Input: part model. Units: mm. Frame: model coordinates. Round coordinates to 2 decimals unless told otherwise and drop trailing zeros. Write each loop counter-clockwise with the first axis right and the second up, starting at its lowest first coordinate (ties: lowest second). Pieces come first, ordered by that corner, then holes. Notation, with made-up numbers: (36.5, -40) -> (66.5, -40) arc R14 cw to (66.5, -32) -> close; hole circle Ø9 at (85, 84.25). An arc over 180 degrees is marked (long way). Write item = value, one per line. Start each with the question number.
```python
from build123d import *

# Parameters (mm, degrees)
SKETCH1_W           = 108.65
SKETCH1_H           = 116
BOSS_EXTRUDE1_DEPTH = 4
SKETCH2_R           = 9
CUT_EXTRUDE1_DEPTH  = 80.568873468
SKETCH4_R           = 2
CUT_EXTRUDE2_DEPTH  = 80.568873468


with BuildPart() as part:
    # Sketch1 → Boss-Extrude1 (new body)
    with BuildSketch(Plane.XY):
        Rectangle(SKETCH1_W, SKETCH1_H)
    extrude(amount=BOSS_EXTRUDE1_DEPTH)

    # Sketch2 → Cut-Extrude1 (cut, through all)
    with BuildSketch(Plane.XY.offset(4)):
        with Locations((26.325, 37.5)):
            Circle(SKETCH2_R)
        with Locations((-32.175, 32.6)):
            Circle(SKETCH2_R)
    extrude(amount=-CUT_EXTRUDE1_DEPTH, mode=Mode.SUBTRACT)

    # Sketch4 → Cut-Extrude2 (cut, through all)
    with BuildSketch(Plane.XY.offset(4)):
        with Locations((-45.325, 54.5)):
            Circle(SKETCH4_R)
        with Locations(Location((-45.325, -54.5, 0), (0, 0, 180))):
            Circle(SKETCH4_R)
        with Locations(Location((-9.025, 54.5, 0), (0, 0, 180))):
            Circle(SKETCH4_R)
        with Locations((-9.025, -54.5)):
            Circle(SKETCH4_R)
        with Locations(Location((-23.025, -54.5, 0), (0, 0, 180))):
            Circle(SKETCH4_R)
        with Locations((7.475, 54.5)):
            Circle(SKETCH4_R)
        with Locations(Location((7.475, -54.5, 0), (0, 0, 180))):
            Circle(SKETCH4_R)
        with Locations((45.325, 54.5)):
            Circle(SKETCH4_R)
        with Locations(Location((45.325, -54.5, 0), (0, 0, 180))):
            Circle(SKETCH4_R)
    extrude(amount=-CUT_EXTRUDE2_DEPTH, mode=Mode.SUBTRACT)


solid = part.part
```
1. Section A-A (y = -54.5). Output: boundary loops of the cut face in (x, z) (3 decimals), then the cut area to 3 significant figures.
2. Mould query, pull axis Y, two halves, no side actions, for faces 1 (the flat face through (-1, 58, 2)), 2 (the flat face through (-54.325, -1, 2)), 3 (the cylindrical face through (-23.59, 35.3, 2.03)), 4 (the flat face through (-1, -58, 2)). Classes: pulls with the +Y half, pulls with the -Y half, needs draft (parallel to the pull), parting line crosses it, or undercut.
3. Line query: line 1 along X through (y, z) = (40, 0.55) (1 decimal); line 2 along Y through (x, z) = (-47, 2.65); line 3 along Y through (x, z) = (-22, 1.8). Output: solid intervals per line, ascending.
4. Section C-C (y = 54.5). Output: boundary loops of the cut face in (x, z) (3 decimals).
5. Section B-B (z = 1.2). State how many separate pieces and enclosed holes the cut face has, then the cut area to 3 significant figures.
6. Section D-D (x = 25.5). Output: boundary loops of the cut face in (y, z).
7. Pin query (flat end, axial travel): P1, Ø16, axis at x = -32.175, y = 32.6, coming from the -Z side; P2, Ø6.5, axis at x = -23.025, y = -54.5, coming from the +Z side. Return the tip coordinate at first contact, or that it passes through.
Check sheet entries:
q1.outline = (-54.325, 0) -> (-47.325, 0) -> (-47.325, 4) -> (-54.325, 4) -> close; (-43.325, 0) -> (-25.025, 0) -> (-25.025, 4) -> (-43.325, 4) -> close; (-21.025, 0) -> (-11.025, 0) -> (-11.025, 4) -> (-21.025, 4) -> close; (-7.025, 0) -> (5.475, 0) -> (5.475, 4) -> (-7.025, 4) -> close; (9.475, 0) -> (43.325, 0) -> (43.325, 4) -> (9.475, 4) -> close; (47.325, 0) -> (54.325, 0) -> (54.325, 4) -> (47.325, 4) -> close
q1.area = 355 mm2
q2.face_1 = pulls with the +Y half
q2.face_2 = needs draft
q2.face_3 = undercut
q2.face_4 = pulls with the -Y half
q3.line_1 = -54.3 to -37.3, -27.1 to 17.7, 35 to 54.3
q3.line_2 = -58 to -55.59, -53.41 to 53.41, 55.59 to 58
q3.line_3 = -58 to -56.22, -52.78 to 58
q4.outline = (-54.325, 0) -> (-47.325, 0) -> (-47.325, 4) -> (-54.325, 4) -> close; (-43.325, 0) -> (-11.025, 0) -> (-11.025, 4) -> (-43.325, 4) -> close; (-7.025, 0) -> (5.475, 0) -> (5.475, 4) -> (-7.025, 4) -> close; (9.475, 0) -> (43.325, 0) -> (43.325, 4) -> (9.475, 4) -> close; (47.325, 0) -> (54.325, 0) -> (54.325, 4) -> (47.325, 4) -> close
q5.separate_pieces = 1
q5.enclosed_holes = 11
q5.area = 12,000 mm2
q6.outline = (-58, 0) -> (28.54, 0) -> (28.54, 4) -> (-58, 4) -> close; (46.46, 0) -> (58, 0) -> (58, 4) -> (46.46, 4) -> close
q7.P1 = through
q7.P2 = 4
